Autodesk Fusion 360 part; units mm, degrees
sketch "Skizze1" plane through (0, 0, 0) normal (0, 0, 1) x (1, 0, 0)
  circle A0 centre (0, 0) radius 10
  circle A1 centre (0, 0) radius 9.25
  circle A2 centre (0, 0) radius 3.95
  circle A3 centre (0, 0) radius 10.85
  dimension "d1" = 20
  dimension "d2" = -0.75
  dimension "d3" = 7.9
  dimension "d4" = 1.6
extrude "Extrusion1" add sketch "Skizze1" along normal blind 8.5 contours A0 | A1 | A2
sketch "Skizze4" plane through (0, 0, 8.5) normal (0, 0, 1) x (-1, 0, 0)
  circle A0 centre (0, 0) radius 10
  circle A1 centre (0, 0) radius 2.525
  circle A2 centre (0, 0) radius 3.5
  dimension "d20" = 5.05
  dimension "d21" = 7
extrude "Extrusion5" add sketch "Skizze1" along normal blind 8.5 contours A3
extrude "Extrusion6" cut sketch "Skizze1" along normal blind 7.5 contours A3
extrude "Extrusion8" add sketch "Skizze4" along normal blind 9.7 contours A1
extrude "Extrusion9" add sketch "Skizze4" along normal blind 2.5 contours A2
sketch "Skizze5" plane through (0, 0, 18.2) normal (0, 0, 1) x (-1, 0, 0)
  circle A0 centre (0, 0) radius 2.525
  circle A1 centre (0, 0) radius 0.9
  dimension "d27" = 1.8
extrude "Extrusion10" cut sketch "Skizze5" against normal blind 21 contours A1
equation "d5 = 11 mm - 2.5 mm"
equation "d14 = 11 mm - 2.5 mm"
equation "d16 = 10 mm - 2.5 mm"
Work out the finished part from the listing and answer in its coordinate system (mm). A direction names the side the tool comes from. Round coordinates to 2 decimals unless told otherwise and drop trailing zeros. Loops run counter-clockwise (first coordinate to the right, second up) from the corner with the lowest first, then second, coordinate; pieces in that order, holes last.
(1) The part is cut by section A-A, the plane x = -0.5. Give the vertices of the cut face in (y, z) (1 decimal), and give its area (3 significant figures).
Computed values:
outline: (-10.8, 7.5) - (-10, 7.5) - (-10, 0) - (-0.7, 0) - (-0.7, 18.2) - (-2.5, 18.2) - (-2.5, 11) - (-3.5, 11) - (-3.5, 8.5) - (-10.8, 8.5) - close; (0.7, 0) - (10, 0) - (10, 7.5) - (10.8, 7.5) - (10.8, 8.5) - (3.5, 8.5) - (3.5, 11) - (2.5, 11) - (2.5, 18.2) - (0.7, 18.2) - close
area: 197 mm2
(2) The part is cut by section C-C, the plane x = 5.75. Give the vertices of the cut face in (y, z), and give its area (3 significant figures).
Computed values:
outline: (-9.2, 7.5) - (-8.18, 7.5) - (-8.18, 0) - (8.18, 0) - (8.18, 7.5) - (9.2, 7.5) - (9.2, 8.5) - (-9.2, 8.5) - close
area: 141 mm2
(3) For faces 1 (the cylindrical face through (-3.233, -1.341, 9.732)), 2 (the flat face through (-1.1, 0, 18.2)), 3 (the cylindrical face through (-2.17, 9.76, 3.7)), determine the directions among +Z, -Z, +X, -X, +Y, -Y from which every point of the face is accessible in a straight line to the end or side of a thin tool.
Computed values:
face 1: +Z
face 2: +Z, +X, -X, +Y, -Y
face 3: -Z
(4) The part is cut by section B-B, the plane z = 14. Give the vertices of the cut face in (x, y) (3 decimals), and give its area (3 significant figures).
Computed values:
outline: circle Ø5.05 at (0, 0); hole circle Ø1.8 at (0, 0)
area: 17.5 mm2
(5) Find the intervals of material crossed by L1, parallel to X at y = 0, z = 13.25 (3 decimals); L2, parallel to X at y = 0, z = 9.25, in increasing order.
Computed values:
L1: x = -2.525 to -0.9, 0.9 to 2.525
L2: x = -3.5 to -0.9, 0.9 to 3.5
(6) The part is cut by section D-D, the plane y = 1.5. Give the vertices of the cut face in (x, z).
Computed values:
outline: (-10.75, 7.5) - (-9.89, 7.5) - (-9.89, 0) - (9.89, 0) - (9.89, 7.5) - (10.75, 7.5) - (10.75, 8.5) - (3.16, 8.5) - (3.16, 11) - (2.03, 11) - (2.03, 18.2) - (-2.03, 18.2) - (-2.03, 11) - (-3.16, 11) - (-3.16, 8.5) - (-10.75, 8.5) - close
(7) The mould has two halves that part along Y. Classify faces 4 (the flat face through (-3, 3, 8.5)), 5 (the cylindrical face through (-8, -7.33, 7.99)), 6 (the cylindrical face through (-0.86, -0.27, 9.23)): pulls with the +Y half, pulls with the -Y half, needs draft (parallel to the pull), parting line crosses it, or undercut.
Computed values:
face 4: needs draft
face 5: parting line crosses it
face 6: undercut
(8) Each of these flat-tipped pins is pushed along its axis until it touches: P1, Ø4, axis at x = 4, z = 2, coming from the +Y side; P2, Ø1, axis at x = 6, z = 2, coming from the +Y side; P3, Ø2, axis at x = -2.5, z = 10, coming from the +Y side. Where does it stop, or does it pass through?
Computed values:
P1: stops at y = 9.8
P2: stops at y = 8.35
P3: stops at y = 3.16
